Design review of the part built by this model. Coordinates are the model's own, in mm. A direction names the side the tool comes from. Round coordinates to 2 decimals unless told otherwise and drop trailing zeros. Loops run counter-clockwise (first coordinate to the right, second up) from the corner with the lowest first, then second, coordinate; pieces in that order, holes last. Notation, with made-up numbers: M -25.75,23.5 L 10.25,23.5 A19 ccw 10.25,58.5 Z; hole C 52.25,77 d1. An arc over 180 degrees is marked long. Use a Markdown table: item, result.
from build123d import *

# Parameters (mm, degrees)
SKETCH_1_W             = 16
SKETCH_1_H             = 16
EXTRUDE_1_DEPTH        = 80
SKETCH_2_R             = 5.75
CUT_EXTRUDE_1_DEPTH    = 50
SKETCH_10_W            = 12
SKETCH_10_H            = 8
SKETCH_10_H_2          = 3
CUT_EXTRUDE_2_DEPTH    = 10
SKETCH_11_R            = 3.25
CUT_EXTRUDE_5_DEPTH    = 1
HOLE_WIZARD_M4_1_D     = 3.3
HOLE_WIZARD_M4_1_DEPTH = 4


with BuildPart() as part:
    # 草图1 → 凸台-拉伸1 (new body)
    with BuildSketch(Plane.XY):
        with Locations((8, -8)):
            Rectangle(SKETCH_1_W, SKETCH_1_H)
    extrude(amount=EXTRUDE_1_DEPTH)

    # 草图2 → 切除-拉伸1 (cut)
    with BuildSketch(Plane.XY.offset(80)):
        with Locations((8, -8)):
            Circle(SKETCH_2_R)
    extrude(amount=-CUT_EXTRUDE_1_DEPTH, mode=Mode.SUBTRACT)

    # 草图10 → 切除-拉伸2 (cut)
    with BuildSketch(Plane(origin=(0, 0, 0), x_dir=(-1, 0, 0), z_dir=(0, 0, -1))):
        with Locations((-8, -4)):
            Rectangle(SKETCH_10_W, SKETCH_10_H)
        with Locations((-8, -14.5)):
            Rectangle(SKETCH_10_W, SKETCH_10_H_2)
    extrude(amount=-CUT_EXTRUDE_2_DEPTH, mode=Mode.SUBTRACT)

    # 草图11 → 切除-拉伸5 (cut)
    with BuildSketch(Plane.XZ.offset(13)):
        with Locations((8, 5)):
            Circle(SKETCH_11_R)
    extrude(amount=-CUT_EXTRUDE_5_DEPTH, mode=Mode.SUBTRACT)

    # M4 螺纹孔的螺纹孔钻头1
    with Locations(Plane(origin=(0, -12, 0), x_dir=(-1, 0, 0), z_dir=(0, -1, 0))):
        with Locations((-8, -5)):
            Hole(HOLE_WIZARD_M4_1_D / 2, depth=HOLE_WIZARD_M4_1_DEPTH)


solid = part.part
1. Take a section at B-B on z = 5. Give the boundary of the cut face in (x, y).
Check values:
| item | result |
|---|---|
| outline | M 0,-16 L 2,-16 L 2,-13 L 4.75,-13 L 4.75,-12 L 6.35,-12 L 6.35,-8 L 2,-8 L 2,0 L 0,0 Z; M 9.65,-12 L 11.25,-12 L 11.25,-13 L 14,-13 L 14,-16 L 16,-16 L 16,0 L 14,0 L 14,-8 L 9.65,-8 Z |
2. The part is to be moulded in two halves that separate along X. For faces 4 (the face through (8, -10, 0)), 5 (the face through (0, -8, 39)), 6 (the face through (9.4, -8, 3.8)), say which applies: pulls with the +X half, pulls with the -X half, needs draft (parallel to the pull), parting line crosses it, or undercut.
Check values:
| item | result |
|---|---|
| face 4 | needs draft |
| face 5 | pulls with the -X half |
| face 6 | undercut |
3. Insertion check: pin 1 (3 mm diameter, centred on x = 10, z = 7, fed in from -Y); pin 2 (7.5 mm diameter, centred on x = 8, z = 5, fed in from +Y); pin 3 (6 mm diameter, centred on x = 9, y = -6, fed in from +Z). Each pin has a flat end and moves straight along its axis. Give the tip position at first contact, or say it passes through.
Check values:
| item | result |
|---|---|
| pin 1 | stops at y = -13 |
| pin 2 | stops at y = -8 |
| pin 3 | stops at z = 30 |
4. Take a section at A-A on x = 8. Give the boundary of the cut face in (y, z), and give its area (3 significant figures).
Check values:
| item | result |
|---|---|
| outline | M -16,10 L -13,10 L -13,8.25 L -12,8.25 L -12,6.65 L -8,6.65 L -8,10 L 0,10 L 0,80 L -2.25,80 L -2.25,30 L -13.75,30 L -13.75,80 L -16,80 Z; M -13,0 L -8,0 L -8,3.35 L -12,3.35 L -12,1.75 L -13,1.75 Z |
| area | 575 mm² |
5. Machinability: for faces 1 (the face through (4.753, -12.507, 5.143)), 2 (the face through (14, -15, 5)), 3 (the face through (8, -8, 30)), which of the approach directions +Z, -Z, +X, -X, +Y, -Y give a long, thin tool a straight path to every point of the face, cutting with its end or side? Answer none if there is none.
Check values:
| item | result |
|---|---|
| face 1 | -Y |
| face 2 | -Z, -Y |
| face 3 | +Z |
6. Take a section at C-C on z = 41. Give the boundary of the cut face in (x, y), and give its area (3 significant figures).
Check values:
| item | result |
|---|---|
| outline | M 0,-16 L 16,-16 L 16,0 L 0,0 Z; hole C 8,-8 d11.5 |
| area | 152 mm² |
7. Wall thickness on line 1 along Z through (x, y) = (8, -12.7); line 2 along Y through (x, z) = (6.25, 49); line 3 along X through (y, z) = (-11, 6): over which ranges is each line inside the solid? List them lowest first. Write a range as from..to.
Check values:
| item | result |
|---|---|
| line 1 | z = 0..1.75, 8.25..30 |
| line 2 | y = -16..-13.48, -2.52..0 |
| line 3 | x = 0..6.69, 9.31..16 |
8. Take a section at D-D on y = -5.5. Give the boundary of the cut face in (x, z), and give its area (3 significant figures).
Check values:
| item | result |
|---|---|
| outline | M 0,0 L 2,0 L 2,10 L 14,10 L 14,0 L 16,0 L 16,80 L 13.18,80 L 13.18,30 L 2.82,30 L 2.82,80 L 0,80 Z |
| area | 642 mm² |
